```python
from build123d import *

# Parameters (mm, degrees)
SWEEP1_START               = -6
SWEEP1_DEPTH               = 12
SKETCH3_R                  = 3
CUT_EXTRUDE1_DEPTH         = 93.552687831
F_3_5_3_5_DIAMETER_HOLE1_D = 3.5
FILLET2_R                  = 2


# Read off the part's stored shape, not the designer's step: Sweep1
with BuildPart() as part:
    # Sweep1 outline → Sweep1 (new body)
    with BuildSketch(Plane.YZ.offset(SWEEP1_START)):
        with BuildLine():
            add(Edge.make_bspline(
                [(0, 6), (31.090204345, 9.606991211), (61.090204345, 17.940324544), (90, 31)],
                knots=[0, 0, 0, 0, 1, 1, 1, 1], degree=3))
            Line((0, 6), (0, -6))
            add(Edge.make_bspline(
                [(0, -6), (31.090204345, -2.393008789), (61.090204345, 5.940324544), (90, 19)],
                knots=[0, 0, 0, 0, 1, 1, 1, 1], degree=3))
            Line((90, 19), (90, 31))
        make_face()
    extrude(amount=SWEEP1_DEPTH)

    # Sketch3 → Cut-Extrude1 (cut, through all)
    with BuildSketch(Plane(origin=(0, 87, 0), x_dir=(1, 0, 0), z_dir=(0, 1, 0))):
        with Locations(Location((0, -25, 0), (0, 0, 270))):
            Circle(SKETCH3_R)
    extrude(amount=-CUT_EXTRUDE1_DEPTH, mode=Mode.SUBTRACT)

    # Ø3.5 (3.5) Diameter Hole1 (through all)
    with Locations(Plane(origin=(0, 87, 0), x_dir=(-1, 0, 0), z_dir=(0, -1, 0))):
        with Locations((0, -25)):
            Hole(F_3_5_3_5_DIAMETER_HOLE1_D / 2)

    # Fillet2
    fillet2_edges = [part.edges().sort_by_distance(p)[0] for p in [
        (6, 45.971752724, 14.998093053),
        (6, 45.971752724, 2.998093053),
        (-6, 45.971752724, 2.998093053),
        (-6, 45.971752724, 14.998093053),
    ]]
    fillet(fillet2_edges, radius=FILLET2_R)


solid = part.part
```
Could you check a few things on this model? Use its own coordinates, in mm. A direction names the side the tool comes from. Round coordinates to 2 decimals unless told otherwise and drop trailing zeros. Answer in a Markdown table with one row per item. Add a question column.
(1) If we mould it in two halves opening along X, with no side actions, what happens to faces 3 (the face through (-2, 87, 25)), 4 (the face through (6, 45, 10)), 5 (the face through (0, 0, 0))? For each: pulls with the +X half, pulls with the -X half, needs draft (parallel to the pull), parting line crosses it, or undercut.
(2) I'm going to push flat-ended pins straight in: pin 1 (4.5 mm diameter, centred on x = 0, z = 25, fed in from -Y); pin 2 (1 mm diameter, centred on x = -2.5, z = 14, fed in from +Y); pin 3 (4 mm diameter, centred on x = 4, y = 68, fed in from -Z). Where does each tip first touch, or does it pass through?
(3) For faces 1 (the face through (-0.228, 88.521, 23.265)), 2 (the face through (0, 80, 22)), which set-ups out of +Z, -Z, +X, -X, +Y, -Y let a thin tool reach every point of the face, with its end or its side?
(4) I need wall thicknesses on line 1 along X through (y, z) = (89.05, 25); line 2 along Y through (x, z) = (-2, 26); line 3 along X through (y, z) = (81.5, 26.5). Which ranges of each line are inside material? Lowest first, please.
Model answer:
| question | item | result |
|---|---|---|
| 1 | face 3 | undercut |
| 1 | face 4 | pulls with the +X half |
| 1 | face 5 | needs draft |
| 2 | pin 1 | stops at y = 87 |
| 2 | pin 2 | stops at y = 79.54 |
| 2 | pin 3 | stops at z = 9.33 |
| 3 | face 1 | +Y, -Y |
| 3 | face 2 | -Y |
| 4 | line 1 | x = -6 to -1.75, 1.75 to 6 |
| 4 | line 2 | y = 87 to 90 |
| 4 | line 3 | x = -5.56 to -2.6, 2.6 to 5.56 |
